Source: CAD feature listing. Evaluate the final solid. Frame: model axes, mm. Give positions to 0.01 mm unless a question says otherwise; leave off trailing zeros. Loops run counter-clockwise (first coordinate to the right, second up) from the corner with the lowest first, then second, coordinate; pieces in that order, holes last.
```python
from build123d import *

# Parameters (mm, degrees)
BOSS_EXTRUDE1_DEPTH = 9
SKETCH2_R           = 1.8
CUT_EXTRUDE1_DEPTH  = 11.5
SHELL1_T            = -1
FILLET3_R           = 3
SKETCH5_R           = 1.65
CUT_EXTRUDE4_DEPTH  = 16
SKETCH6_W           = 5.761789727
SKETCH6_H           = 7.4
CUT_EXTRUDE5_DEPTH  = 3


with BuildPart() as part:
    # Sketch1 → Boss-Extrude1 (new body)
    with BuildSketch(Plane(origin=(-8.550148724, 0.150483818, 31.909921865), x_dir=(0.9659203418587706, 0.0049942121419566075, 0.2587913271895271), z_dir=(-0.2588138443395903, 0.004555159989206847, 0.96591647904756))):
        Polygon((-2.116672777, -0.00038458), (-5.116672777, -0.00038458), (-5.208111757, 9.999197357), (-4.549568011, 13.944614969), (-4.549568011, 103.944614969), (4.716222456, 103.944614969), (4.716222456, 13.944614969), (5.374766202, 9.999197357), (5.283327223, -0.00038458), (2.283327223, -0.00038458), (2.283327223, 8.99961542), (-2.116672777, 8.99961542), align=None)
    extrude(amount=-BOSS_EXTRUDE1_DEPTH)

    # Sketch2 → Cut-Extrude1 (cut, symmetric)
    with BuildSketch(Plane(origin=(-2.044537293, -0.010571113, -0.547776557), x_dir=(0.2588168701543083, -0.005411250453060186, -0.9659112516644903), z_dir=(0.9659203418587706, 0.0049942121419806335, 0.2587913271895269))):
        with Locations(Location((-28.539422387, 4.100183989, 0), (0, 0, 180.310047193))):
            Circle(SKETCH2_R)
    extrude(amount=CUT_EXTRUDE1_DEPTH, both=True, mode=Mode.SUBTRACT)

    # Shell1
    shell1_openings = [part.faces().sort_by_distance(p)[0] for p in [
        (-6.334444908, 53.359699464, 22.935106903),
    ]]
    offset(amount=SHELL1_T, openings=shell1_openings, kind=Kind.INTERSECTION)

    # Fillet3
    # the kernel refuses this fillet: 3 mm, written as the material it takes off along each edge
    with BuildSketch(Plane(origin=(-3.35028205, 0.176984725, 33.303082451), x_dir=(0.2588138443395903, -0.004555159989206649, -0.9659164790475598), z_dir=(-0.9659203418587717, -0.004994212141671299, -0.25879132718952874))) as fillet3_piece_1:
        with BuildLine():
            CenterArc((FILLET3_R, -FILLET3_R), FILLET3_R, 90, 90)
            Line((0, -FILLET3_R), (0, 0))
            Line((0, 0), (FILLET3_R, 0))
        make_face()
    extrude(amount=18, mode=Mode.SUBTRACT)
    with BuildSketch(Plane(origin=(-1.020957451, 0.135988285, 24.609834139), x_dir=(-0.25881384433959026, 0.004555159989206952, 0.9659164790475598), z_dir=(-0.9659203418587717, -0.004994212141671299, -0.25879132718952874)), Plane(origin=(6.126853079, 0.172945455, 26.52488996), x_dir=(-0.25881384433959026, 0.004555159989206913, 0.9659164790475598), z_dir=(-0.9659203418587694, -0.004994212142289673, -0.2587913271895252)), Plane(origin=(3.797528479, 0.213941895, 35.218138272), x_dir=(-0.0036451559089296618, 0.9999771539203036, -0.005692492937989095), z_dir=(-0.9659203418587694, -0.004994212142289673, -0.2587913271895252))) as fillet3_piece_2:
        with BuildLine():
            CenterArc((FILLET3_R, FILLET3_R), FILLET3_R, 180, 90)
            Line((0, FILLET3_R), (0, 0))
            Line((0, 0), (FILLET3_R, 0))
        make_face()
    extrude(amount=18, mode=Mode.SUBTRACT)

    # Sketch5 → Cut-Extrude4 (cut)
    with BuildSketch(Plane(origin=(4.555495207, 0.023553815, 1.220517469), x_dir=(0.2587878680955358, 0.0013380415103731802, -0.9659332528552292), z_dir=(0.9659203418587695, 0.0049942121422931664, 0.25879132718952524))):
        with Locations(Location((-27.180645186, 35.235580785, 0), (0, 0, 359.92333489))):
            Circle(SKETCH5_R)
    extrude(amount=-CUT_EXTRUDE4_DEPTH, mode=Mode.SUBTRACT)

    # Sketch6 → Cut-Extrude5 (cut)
    with BuildSketch(Plane(origin=(-8.550148724, 0.150483818, 31.909921865), x_dir=(0.9659272198142892, 0.0012205251536603987, 0.25881096642180224), z_dir=(-0.2588138443395908, 0.0045551599892071715, 0.9659164790475597))):
        with Locations((-0.252081359, 92.845441705)):
            Rectangle(SKETCH6_W, SKETCH6_H)
    extrude(amount=-CUT_EXTRUDE5_DEPTH, mode=Mode.SUBTRACT)


solid = part.part
```
(1) Mould query, pull axis Y, two halves, no side actions, for faces 1 (the cylindrical face through (-2.859, 0.695, 25.411)), 2 (the flat face through (-12.16, 12.05, 26.29)). Classes: pulls with the +Y half, pulls with the -Y half, needs draft (parallel to the pull), parting line crosses it, or undercut.
A:
face 1: pulls with the -Y half
face 2: undercut
(2) Ray query, line 1 along Y through (x, z) = (-6, 24.25); line 2 along X through (y, z) = (10, 28.25); line 3 along X through (y, z) = (18, 24.5). Return the intervals inside material, ascending.
A:
line 1: y = 9.12 to 10.12, 103.06 to 104.06
line 2: x = -13.01 to -11.98, -10.85 to -4.22, -3.09 to -2.06
line 3: x = -11.37 to -10.33, -2.81 to -1.77
(3) Section B-B, the plane y = 85. Return the cut outline in (x, z).
A:
outline: (-13.25, 30.25) - (-10.92, 21.56) - (-9.96, 21.81) - (-12.03, 29.54) - (-5.01, 31.42) - (-2.94, 23.7) - (-1.97, 23.95) - (-4.3, 32.65) - close
(4) Section A-A, the plane x = -7.25. Return the cut outline in (y, z).
A:
outline: (9.1, 22.9) - (10.1, 22.89) - (10.15, 31.18) - (89.29, 30.8) - (89.3, 31.84) - (9.16, 32.22) - close; (96.69, 30.77) - (103.1, 30.74) - (103.05, 22.46) - (104.05, 22.45) - (104.1, 31.77) - (96.7, 31.8) - close
(5) First-contact query: pin 1 (1.5 mm diameter, centred on x = -2.5, z = 29, fed in from -Y); pin 2 (3 mm diameter, centred on y = 79, z = 25.5, fed in from -X); pin 3 (2 mm diameter, centred on x = -3, z = 27.5, fed in from -Y). Flat tips, straight axial feed; report the tip coordinate or a pass-through.
A:
pin 1: stops at y = 0.15
pin 2: stops at x = -12.35
pin 3: stops at y = 0.14
